Verification items for the finished model (mm, model axes). A direction names the side the tool comes from. Give positions to 0.01 mm unless a question says otherwise; leave off trailing zeros. Write each loop counter-clockwise with the first axis right and the second up, starting at its lowest first coordinate (ties: lowest second). Pieces come first, ordered by that corner, then holes. Notation, with made-up numbers: (74.25, 41.25) -> (115.25, 41.25) arc R19 cw to (115.25, 56.25) -> close; hole circle Ø8 at (43, 46.25). An arc over 180 degrees is marked (long way). Write item = value, one per line.
from build123d import *

# Parameters (mm, degrees)
SKETCH_1_R               = 18
EXTRUDE_1_DEPTH          = 72
EXTRUDE_2_DEPTH          = 25
EXTRUDE_2_DEPTH_BACK     = 25
SKETCH_2_R               = 24.5
CUT_EXTRUDE_1_DEPTH      = 101.669012284
SKETCH_5_R               = 8.5
EXTRUDE_3_DEPTH          = 6
CUT_EXTRUDE_2_DEPTH      = 10
CUT_EXTRUDE_2_DEPTH_BACK = 12
EXTRUDE_START            = -10.5
EXTRUDE_4_DEPTH          = 10.5
SKETCH_7_R               = 2.5
CUT_EXTRUDE_3_DEPTH      = 5


with BuildPart() as part:
    # Sketch 1 → Extrude 1 (new body)
    with BuildSketch(Plane(origin=(0, 0, 0), x_dir=(1, 0, 0), z_dir=(0, 1, 0))):
        with Locations(Location((0, 0, 0), (0, 0, 270))):
            Circle(SKETCH_1_R)
    extrude(amount=EXTRUDE_1_DEPTH)

    # Sketch 2 → Extrude 2 (add, two sides: drawn at the far end of the back side and taken through both)
    with BuildSketch(Plane(origin=(0, 0, 0), x_dir=(0, 0, -1), z_dir=(1, 0, 0)).offset(-EXTRUDE_2_DEPTH_BACK)):
        with Locations((25, 36)):
            Circle(SKETCH_2_R)
    extrude(amount=EXTRUDE_2_DEPTH + EXTRUDE_2_DEPTH_BACK)

    # Sketch 3 → Cut-Extrude 1 (cut, through all)
    with BuildSketch(Plane(origin=(25, 0, 0), x_dir=(0, 0, -1), z_dir=(1, 0, 0))):
        with BuildLine():
            Line((23, 41.123475383), (23, 43))
            Line((23, 43), (27, 43))
            Line((27, 43), (27, 41.123475383))
            ThreePointArc((27, 41.123475383), (25, 30.5), (23, 41.123475383))
        make_face()
    extrude(amount=-CUT_EXTRUDE_1_DEPTH, mode=Mode.SUBTRACT)

    # Sketch 5 → Extrude 3 (add)
    with BuildSketch(Plane(origin=(0, 72, 0), x_dir=(1, 0, 0), z_dir=(0, 1, 0))):
        with Locations(Location((0, 0, 0), (0, 0, 270))):
            Circle(SKETCH_5_R)
    extrude(amount=EXTRUDE_3_DEPTH)

    # Sketch 4 → Cut-Extrude 2 (cut, two sides: drawn at the far end of the back side and taken through both)
    with BuildSketch(Plane(origin=(0, 72, 0), x_dir=(1, 0, 0), z_dir=(0, 1, 0)).offset(-CUT_EXTRUDE_2_DEPTH_BACK)):
        with BuildLine():
            Line((-1.5, -4.242640687), (-1.5, -6.5))
            Line((-1.5, -6.5), (1.5, -6.5))
            Line((1.5, -6.5), (1.5, -4.242640687))
            ThreePointArc((1.5, -4.242640687), (0, 4.5), (-1.5, -4.242640687))
        make_face()
    extrude(amount=CUT_EXTRUDE_2_DEPTH + CUT_EXTRUDE_2_DEPTH_BACK, mode=Mode.SUBTRACT)

    # Sketch 6 → Extrude 4 (add)
    with BuildSketch(Plane(origin=(0, 72, 0), x_dir=(1, 0, 0), z_dir=(0, 1, 0)).offset(EXTRUDE_START)):
        with BuildLine():
            Line((-20.668584287, 10.200961894), (-19.168584287, 12.799038106))
            ThreePointArc((-19.168584287, 12.799038106), (-17.346965211, 14.196815585), (-15.070508076, 13.897114317))
            Line((-15.070508076, 13.897114317), (-12.843458848, 12.611326846))
            ThreePointArc((-12.843458848, 12.611326846), (-15.588457268, 9), (-17.343458848, 4.817098212))
            Line((-17.343458848, 4.817098212), (-19.570508076, 6.102885683))
            ThreePointArc((-19.570508076, 6.102885683), (-20.968285555, 7.924504759), (-20.668584287, 10.200961894))
        make_face()
        with BuildLine():
            Line((1.5, -23), (-1.5, -23))
            ThreePointArc((-1.5, -23), (-3.621320344, -22.121320344), (-4.5, -20))
            Line((-4.5, -20), (-4.5, -17.428425058))
            ThreePointArc((-4.5, -17.428425058), (0, -18), (4.5, -17.428425058))
            Line((4.5, -17.428425058), (4.5, -20))
            ThreePointArc((4.5, -20), (3.621320344, -22.121320344), (1.5, -23))
        make_face()
        with BuildLine():
            Line((19.168584287, 12.799038106), (20.668584287, 10.200961894))
            ThreePointArc((20.668584287, 10.200961894), (20.968285555, 7.924504759), (19.570508076, 6.102885683))
            Line((19.570508076, 6.102885683), (17.343458848, 4.817098212))
            ThreePointArc((17.343458848, 4.817098212), (15.588457268, 9), (12.843458848, 12.611326846))
            Line((12.843458848, 12.611326846), (15.070508076, 13.897114317))
            ThreePointArc((15.070508076, 13.897114317), (17.346965211, 14.196815585), (19.168584287, 12.799038106))
        make_face()
    extrude(amount=EXTRUDE_4_DEPTH)

    # Sketch 7 → Cut-Extrude 3 (cut)
    with BuildSketch(Plane(origin=(0, 72, 0), x_dir=(1, 0, 0), z_dir=(0, 1, 0))):
        with Locations(Location((0, -19, 0), (0, 0, 270))):
            Circle(SKETCH_7_R)
        with Locations(Location((16.454482672, 9.5, 0), (0, 0, 270))):
            Circle(SKETCH_7_R)
        with Locations(Location((-16.454482672, 9.5, 0), (0, 0, 270))):
            Circle(SKETCH_7_R)
    extrude(amount=-CUT_EXTRUDE_3_DEPTH, mode=Mode.SUBTRACT)


solid = part.part
Item 1: Sectioned sample at B-B on y = 39. Record the cut outline in (x, z).
Response values:
outline = (-25, -49.32) -> (25, -49.32) -> (25, -29.61) -> (-25, -29.61) -> close; (-25, -20.39) -> (25, -20.39) -> (25, -0.68) -> (17.99, -0.68) arc R18 ccw (long way) to (-17.99, -0.68) -> (-25, -0.68) -> close
Item 2: Sectioned sample at C-C on x = 6.5. Record the cut outline in (y, z).
Response values:
outline = (0, -16.79) -> (12.92, -16.79) arc R24.5 ccw (long way) to (59.08, -16.79) -> (72, -16.79) -> (72, -5.48) -> (78, -5.48) -> (78, 5.48) -> (72, 5.48) -> (72, 16.79) -> (0, 16.79) -> close; hole (41.12, -27) -> (43, -27) -> (43, -23) -> (41.12, -23) arc R5.5 ccw (long way) to start
Item 3: Sectioned sample at A-A on z = -25. Record the cut outline in (x, y).
Response values:
outline = (-25, 11.5) -> (25, 11.5) -> (25, 30.5) -> (-25, 30.5) -> close; (-25, 43) -> (25, 43) -> (25, 60.5) -> (-25, 60.5) -> close
Item 4: Go/stop test with flat-tipped pins: P1, Ø1, axis at x = -11.5, y = 28, coming from the -Z side; P2, Ø2, axis at x = -9, y = 67, coming from the -Z side; P3, Ø2, axis at x = 1.5, z = -25.5, coming from the -Y side; P4, Ø6.5, axis at y = 36, z = -25, coming from the +X side. Record where each tip stops, or that it passes through.
Response values:
P1 = -48.32
P2 = -16.12
P3 = 11.5
P4 = through
Item 5: Sectioned sample at D-D on z = 19. Record the cut outline in (x, y).
Response values:
outline = (-4.5, 61.5) -> (4.5, 61.5) -> (4.5, 72) -> (2.5, 72) -> (2.5, 67) -> (-2.5, 67) -> (-2.5, 72) -> (-4.5, 72) -> close
Item 6: Mould release check, pull along Y, two halves, no side actions. Record for faces 5 (the cylindrical face through (0.176, 68.874, -4.497)), 6 (the flat face through (0, 43, -25)): +Y half, -Y half, draft (parallel to the pull), parting line (faces both ways), or undercut.
Response values:
face_5 = draft
face_6 = undercut
Item 7: Material ranges on line 1 (X direction, y = 70, z = 19); line 2 (X direction, y = 69, z = 0); line 3 (X direction, y = 68.15, z = -9.5), recorded low to high.
Response values:
line_1 = -4.5 to -2.5, 2.5 to 4.5
line_2 = -18 to -4.5, 4.5 to 18
line_3 = -20.96 to -18.95, -13.95 to 13.95, 18.95 to 20.96
Item 8: Set-up check for faces 1 (the flat face through (13.941, 66.676, -13.245)), 2 (the cylindrical face through (5.407, 35.496, 17.169)), 3 (the cylindrical face through (20.977, 66.676, -7.956)), 4 (the flat face through (0, 42, -23)): record each of +Z, -Z, +X, -X, +Y, -Y from which the full face is reachable in a straight line by a thin tool's end or side.
Response values:
face_1 = -Z, +Y
face_2 = none
face_3 = +X, +Y
face_4 = +X, -X
